```python
from build123d import *

# Parameters (mm, degrees)
BOSS_EXTRUDE1_DEPTH     = 1
SKETCH4_W               = 5
SKETCH4_H               = 10
BOSS_EXTRUDE2_DEPTH     = 0.5
CUT_EXTRUDE2_DEPTH      = 19.842742091
CUT_EXTRUDE2_DEPTH_BACK = 19.842742091
SKETCH3_R               = 2
FILLET1_SIZE            = 1


with BuildPart() as part:
    # Sketch1 → Boss-Extrude1 (new body)
    with BuildSketch(Plane.XY):
        with BuildLine():
            Line((-3, -6.860294118), (3, -6.860294118))
            ThreePointArc((3, -6.860294118), (4.414213562, -6.27450768), (5, -4.860294118))
            Line((5, -4.860294118), (5, 3.139705882))
            Line((5, 3.139705882), (3.115711504, 17.271869602))
            ThreePointArc((3.115711504, 17.271869602), (2.783208235, 17.89209), (2.124483603, 18.139705882))
            Line((2.124483603, 18.139705882), (-2.124483603, 18.139705882))
            ThreePointArc((-2.124483603, 18.139705882), (-2.783208235, 17.89209), (-3.115711504, 17.271869602))
            Line((-3.115711504, 17.271869602), (-5, 3.139705882))
            Line((-5, 3.139705882), (-5, -4.860294118))
            ThreePointArc((-5, -4.860294118), (-4.414213562, -6.27450768), (-3, -6.860294118))
        make_face()
    extrude(amount=BOSS_EXTRUDE1_DEPTH)

    # Sketch4 → Boss-Extrude2 (add)
    with BuildSketch(Plane.XY.offset(1)):
        with Locations((0, -1.860294118)):
            Rectangle(SKETCH4_W, SKETCH4_H)
    extrude(amount=BOSS_EXTRUDE2_DEPTH)

    # Sketch3 → Cut-Extrude2 (cut, two sides: drawn at the far end of the back side and taken through both)
    with BuildSketch(Plane.XY.offset(1).offset(-CUT_EXTRUDE2_DEPTH_BACK)):
        with Locations((0, -1.860294118)):
            Circle(SKETCH3_R)
    extrude(amount=CUT_EXTRUDE2_DEPTH + CUT_EXTRUDE2_DEPTH_BACK, mode=Mode.SUBTRACT)

    # Sketch10 → Revolve1 (revolve)
    with BuildSketch(Plane.ZY):
        with BuildLine():
            Line((3, 13.139705882), (1, 13.139705882))
            Line((1, 13.139705882), (1, 15.164832594))
            add(Edge.make_bspline(
                [(1, 15.164832594), (1.103472507, 14.776659397), (2.95133834, 14.490964633), (3, 13.139705882)],
                knots=[0, 0, 0, 0, 1, 1, 1, 1], degree=3))
        make_face()
    revolve(axis=Axis((0, 13.139705882, 3), (0, 0, -1)))

    # Fillet1
    # a fillet whose section is not a circle: 1 mm, written as the material it takes off along each edge
    with BuildSketch(Plane(origin=(2.5, 3.139705882, 1), x_dir=(-1, 0, 0), z_dir=(0, 0, 1)), Plane(origin=(-2.5, 3.139705882, 1), x_dir=(0, -1, 0), z_dir=(0, 0, 1))) as fillet1_piece_1:
        with BuildLine():
            add(Edge.make_bspline([(FILLET1_SIZE, 0), (FILLET1_SIZE * 0.831801948466, 0), (FILLET1_SIZE * 0.663603896932, 0), (FILLET1_SIZE * 0.292893218813, FILLET1_SIZE * 0.0716919198361), (FILLET1_SIZE * 0.0716919198361, FILLET1_SIZE * 0.292893218813), (0, FILLET1_SIZE * 0.663603896932), (0, FILLET1_SIZE * 0.831801948466), (0, FILLET1_SIZE)], knots=[0, 0, 0, 0, 0, 0, 0.5, 0.5, 1, 1, 1, 1, 1, 1], degree=5))
            Line((0, FILLET1_SIZE), (0, 0))
            Line((0, 0), (FILLET1_SIZE, 0))
        make_face()
    extrude(amount=3, mode=Mode.SUBTRACT)


solid = part.part
```
Verification items for the finished model (mm, model axes). A direction names the side the tool comes from. Coordinates: 2 decimals unless noted, no trailing zeros. Order: outer loops, then holes, each group sorted by start corner. A loop starts at its lowest first (then second) coordinate and runs counter-clockwise, first axis right, second up. Notation, with made-up numbers: (64, -36) -> (72, -36) arc R31 cw to (72, -4) -> close; hole circle Ø2 at (-10.75, 86). An arc over 180 degrees is marked (long way). Put each result on its own line as item: value. Start each with the question number.
1) Go/stop test with flat-tipped pins: pin 1 (1.5 mm diameter, centred on y = -1, z = 2, fed in from -X); pin 2 (5 mm diameter, centred on x = 0, y = -1.86, fed in from -Z); pin 3 (4 mm diameter, centred on x = -0.5, y = -0.5, fed in from +Z); pin 4 (1.5 mm diameter, centred on x = 3.5, y = 14.5, fed in from +Z). Record where each tip stops, or that it passes through.
2) Tool access check on faces 1 (the flat face through (0, 18.14, 0.5)), 2 (the flat face through (-2, -1, 1.5)). Record the directions out of +Z, -Z, +X, -X, +Y, -Y that give a thin tool (end or side, any length) a straight path to the whole face; none if there is none.
3) Cross-section at C-C (y = 6.5). Enter the section's corners in (x, z), plus the area to 3 significant figures.
4) Cross-section at A-A (z = 1.25). State how many separate pieces and enclosed holes the cut face has, plus the area to 3 significant figures.
5) Cross-section at B-B (x = -4). Enter the section's corners in (y, z), plus the area to 3 significant figures.
6) Material ranges on L1, parallel to X at y = -1.75, z = 0.5; L2, parallel to Y at x = 0, z = 1.15; L3, parallel to Y at x = 0, z = 0.45, recorded low to high.
7) Release check for a two-part mould opening along Y. For faces 3 (the flat face through (-5, -0.8, 0.5)), 4 (the flat face through (0, 6, 1)), 5 (the flat face through (-4.045, 10.305, 0.493)) record: pulls with the +Y half, pulls with the -Y half, needs draft (parallel to the pull), parting line crosses it, or undercut.
Geometry check:
1. pin 1: stops at x = -2.5
1. pin 2: stops at z = 0
1. pin 3: stops at z = 1.5
1. pin 4: stops at z = 1
2. face 1: +Z, -Z, +X, -X, +Y
2. face 2: +Z, +X, -X, -Y
3. outline: (-4.55, 0) -> (4.55, 0) -> (4.55, 1) -> (-4.55, 1) -> close
3. area: 9.10 mm^2
4. separate pieces: 2
4. enclosed holes: 1
4. area: 47.2 mm^2
5. outline: (-6.59, 0) -> (10.64, 0) -> (10.64, 1) -> (-6.59, 1) -> close
5. area: 17.2 mm^2
6. L1: x = -5 to -2, 2 to 5
6. L2: y = -6.86 to -3.86, 0.14 to 3.14, 11.28 to 14.99
6. L3: y = -6.86 to -3.86, 0.14 to 18.14
7. face 3: needs draft
7. face 4: undercut
7. face 5: pulls with the +Y half
